```python
from build123d import *

# Parameters (mm, degrees)
F0_R     = 1.5
F1_DEPTH = 1.5
F2_DEPTH = 9


with BuildPart() as f1:
    # F0 (on Top) → F1 (new body)
    with BuildSketch(Plane.XY):
        with BuildLine():
            ThreePointArc((0, -6.5), (-6.345554, -1.408528), (-2.75012, 5.889554))
            Line((-2.75012, 5.889554), (-25, -4.5))
            Line((-25, -4.5), (-25, -6.5))
            Line((-25, -6.5), (0, -6.5))
        make_face()
        with BuildLine():
            ThreePointArc((0, -6.5), (4.596194, -4.596194), (6.5, 0))
            ThreePointArc((6.5, 0), (3.491004, 5.482964), (-2.75012, 5.889554))
            ThreePointArc((-2.75012, 5.889554), (-6.345554, -1.408528), (0, -6.5))
        make_face()
        with BuildLine():
            ThreePointArc((3.270369, 3.270369), (4.272943, 1.769911), (4.625, 0))
            ThreePointArc((4.625, 0), (4.267428, -1.783168), (3.25, -3.290612))
            ThreePointArc((3.25, -3.290612), (2.112462, -4.114381), (0.780118, -4.558732))
            ThreePointArc((0.780118, -4.558732), (-4.407416, 1.401894), (3.270369, 3.270369))
        make_face(mode=Mode.SUBTRACT)
        with BuildLine():
            ThreePointArc((0.780118, -4.558732), (2.112462, -4.114381), (3.25, -3.290612))
            ThreePointArc((3.25, -3.290612), (3.715891, -1.67444), (3.875, 0))
            ThreePointArc((3.875, 0), (-0.887645, 3.771964), (-3.468335, -1.728085))
            ThreePointArc((-3.468335, -1.728085), (-1.721911, -3.710444), (0.780118, -4.558732))
        make_face()
        Circle(F0_R, mode=Mode.SUBTRACT)
        with BuildLine():
            ThreePointArc((3.25, -3.290612), (4.267428, -1.783168), (4.625, 0))
            ThreePointArc((4.625, 0), (4.272943, 1.769911), (3.270369, 3.270369))
            ThreePointArc((3.270369, 3.270369), (3.724037, 1.663167), (3.875, 0))
            ThreePointArc((3.875, 0), (3.715891, -1.67444), (3.25, -3.290612))
        make_face()
        with BuildLine():
            ThreePointArc((3.875, 0), (3.724037, 1.663167), (3.270369, 3.270369))
            ThreePointArc((3.270369, 3.270369), (-4.407416, 1.401894), (0.780118, -4.558732))
            ThreePointArc((0.780118, -4.558732), (-1.721911, -3.710444), (-3.468335, -1.728085))
            ThreePointArc((-3.468335, -1.728085), (-0.887645, 3.771964), (3.875, 0))
        make_face()
    extrude(amount=F1_DEPTH)

    # F0 (on Top) → F2 (join)
    with BuildSketch(Plane.XY):
        with BuildLine():
            ThreePointArc((0.780118, -4.558732), (2.112462, -4.114381), (3.25, -3.290612))
            ThreePointArc((3.25, -3.290612), (3.715891, -1.67444), (3.875, 0))
            ThreePointArc((3.875, 0), (-0.887645, 3.771964), (-3.468335, -1.728085))
            ThreePointArc((-3.468335, -1.728085), (-1.721911, -3.710444), (0.780118, -4.558732))
        make_face()
        Circle(F0_R, mode=Mode.SUBTRACT)
    extrude(amount=F2_DEPTH)


solid = f1.part
```
Read the model definition and answer for the solid it produces. Units are mm, in the model's axes. A direction names the side the tool comes from. Coordinates: 2 decimals unless noted, no trailing zeros. Write each loop counter-clockwise with the first axis right and the second up, starting at its lowest first coordinate (ties: lowest second). Pieces come first, ordered by that corner, then holes. Notation, with made-up numbers: (74, 43.5) -> (101, 43.5) arc R18 ccw to (101, 50.5) -> close; hole circle Ø11 at (-3, 14.5). An arc over 180 degrees is marked (long way). Return JSON: item names as keys, results as strings.
1. Determine the mould class of faces 4 (the face through (-0.792, 3.793, 5.198)), 5 (the face through (-1.5, 0.07, 4.44)), 6 (the face through (-13.719, 0.768, 0.74)), 7 (the face through (-6, -1, 1.5)) for opening direction X: pulls with the +X half, pulls with the -X half, needs draft (parallel to the pull), parting line crosses it, or undercut.
Found:
{"face 4": "parting line crosses it", "face 5": "undercut", "face 6": "pulls with the -X half", "face 7": "needs draft"}
2. Find the intervals of material crossed by line 1 along Z through (x, y) = (-2, -4); line 2 along Y through (x, z) = (0, 3.25) (3 decimals); line 3 along X through (y, z) = (-3, 5.5), in increasing order. Write a range as from..to.
Found:
{"line 1": "0..1.5", "line 2": "-4.446..-1.5, 1.5..3.875", "line 3": "-2.57..3.36"}
3. A cutting plane is placed at C-C (y = -4). Determine the outline of the cut face in (x, z), and give its area (3 significant figures).
Found:
{"outline": "(-23.93, 0) -> (5.12, 0) -> (5.12, 1.5) -> (2.32, 1.5) -> (2.32, 9) -> (-1.23, 9) -> (-1.23, 1.5) -> (-23.93, 1.5) -> close", "area": "70.2 mm2"}
4. A tool of negligible diameter and unlimited length cuts with its end or side. For faces 1 (the face through (-1.75, -3.69, 5.2)), 2 (the face through (2, 0, 9)), 3 (the face through (2.095, -4.123, 5.198)), from which of +Z, -Z, +X, -X, +Y, -Y can it reach the whole face along a straight path? Write none if from no direction.
Found:
{"face 1": "+Z, -X, -Y", "face 2": "+Z, +X, -X, +Y, -Y", "face 3": "+Z, +X, -Y"}
5. A cutting plane is placed at A-A (z = 4). Determine the outline of the cut face in (x, y) (3 decimals), and give its area (3 significant figures).
Found:
{"outline": "(-3.468, -1.728) arc R5.122 ccw to (0.78, -4.559) arc R4.625 ccw to (3.25, -3.291) arc R9.06 ccw to (3.875, 0) arc R3.875 ccw (long way) to start; hole circle Ø3 at (0, 0)", "area": "44.2 mm2"}
6. A cutting plane is placed at D-D (x = -13.5). Determine the outline of the cut face in (y, z).
Found:
{"outline": "(-6.5, 0) -> (0.87, 0) -> (0.87, 1.5) -> (-6.5, 1.5) -> close"}
7. Each of these flat-tipped pins is pushed along its axis until it touches: P1, Ø3, axis at y = 4, z = 4, coming from the +X side; P2, Ø4, axis at y = 5, z = 6, coming from the -X side; P3, Ø2, axis at y = -2, z = 5.5, coming from the -X side. Where does it stop, or does it pass through?
Found:
{"P1": "x = 2.96", "P2": "x = -2.45", "P3": "x = -3.74"}
8. A cutting plane is placed at B-B (x = 2). Determine the outline of the cut face in (y, z).
Found:
{"outline": "(-6.18, 0) -> (6.18, 0) -> (6.18, 1.5) -> (3.32, 1.5) -> (3.32, 9) -> (-4.17, 9) -> (-4.17, 1.5) -> (-6.18, 1.5) -> close"}
